```python
from build123d import *

# Parameters (mm, degrees)
SKETCH1_R                   = 30
SKETCH1_R_2                 = 15
BOSS_EXTRUDE1_DEPTH         = 17
SKETCH1_3_R                 = 15
CUT_EXTRUDE1_DEPTH          = 15
M6_TAPPED_HOLE1_D           = 5
M6_TAPPED_HOLE1_DEPTH       = 9
M6_TAPPED_HOLE1_CSINK_D     = 6.05
M6_TAPPED_HOLE1_CSINK_ANGLE = 90
M6_TAPPED_HOLE1_TIP         = 1.502151548


with BuildPart() as part:
    # Sketch1 → Boss-Extrude1 (new body)
    with BuildSketch(Plane.XY):
        Circle(SKETCH1_R)
        Circle(SKETCH1_R_2, mode=Mode.SUBTRACT)
        Circle(SKETCH1_R_2)
    extrude(amount=BOSS_EXTRUDE1_DEPTH)

    # Sketch1_3 → Cut-Extrude1 (cut)
    with BuildSketch(Plane.XY):
        Circle(SKETCH1_3_R)
    extrude(amount=CUT_EXTRUDE1_DEPTH, mode=Mode.SUBTRACT)

    # M6 Tapped Hole1
    with Locations(Plane.XY.offset(17)):
        with Locations((0, -22.5), (22.5, 0), (0, 22.5), (-22.5, 0)):
            CounterSinkHole(M6_TAPPED_HOLE1_D / 2, M6_TAPPED_HOLE1_CSINK_D / 2, depth=M6_TAPPED_HOLE1_DEPTH, counter_sink_angle=M6_TAPPED_HOLE1_CSINK_ANGLE)
            with Locations((0, 0, -(M6_TAPPED_HOLE1_DEPTH + M6_TAPPED_HOLE1_TIP / 2))):  # 118° drill point
                Cone(0, M6_TAPPED_HOLE1_D / 2, M6_TAPPED_HOLE1_TIP, mode=Mode.SUBTRACT)


solid = part.part
```
Here's how the part is built. I have some questions about the finished solid (model axes, mm). A direction names the side the tool comes from. Round coordinates to 2 decimals unless told otherwise and drop trailing zeros. Order: outer loops, then holes, each group sorted by start corner. A loop starts at its lowest first (then second) coordinate and runs counter-clockwise, first axis right, second up. Notation, with made-up numbers: M -16.5,-29.5 L 6.5,-29.5 A11 cw 6.5,-16.5 Z; hole C -6.5,13 d8. An arc over 180 degrees is marked long. One line per question, with ' | ' between items.
1) If we mould it in two halves opening along Y, with no side actions, what happens to faces 4 (the face through (-29.97, 1.32, 8.38)), 5 (the face through (0, 0, 17)), 6 (the face through (0.4, -22.67, 6.76)), 7 (the face through (0, -20, 12))? For each: +Y half, -Y half, draft (parallel to the pull), parting line (faces both ways), or undercut.
Working result:
face 4: parting line | face 5: draft | face 6: undercut | face 7: undercut
2) I need wall thicknesses on line 1 along Y through (x, z) = (0, 12); line 2 along Y through (x, z) = (-0.5, 6.25); line 3 along Z through (x, y) = (11, 4). Which ranges of each line are inside material? Lowest first, please.
Working result:
line 1: -30 to -25, -20 to -15, 15 to 20, 25 to 30 | line 2: -30 to -14.99, 14.99 to 30 | line 3: 15 to 17
3) I want a section at B-B, the plane z = 2.25. Write out the boundary of the cut face in (x, y), then the cut area to 3 significant figures.
Working result:
outline: C 0,0 d60; hole C 0,0 d30 | area: 2,120 mm²
4) For pin 1 Ø1.5 at (y, z) = (20, 5.5) entering from +X; pin 2 Ø8 at (x, z) = (9, 4.5) entering from +Y; pin 3 Ø1 at (y, z) = (-14.5, 4) entering from +X, each with a flat end and sliding along its axis, tell me the tip position at first contact or that it passes through.
Working result:
pin 1: x = 23.01 | pin 2: y = 29.58 | pin 3: x = 26.53
5) I want a section at A-A, the plane z = 15.75. Write out the boundary of the cut face in (x, y), then the cut area to 3 significant figures.
Working result:
outline: C 0,0 d60; hole C -22.5,0 d5; hole C 0,-22.5 d5; hole C 0,22.5 d5; hole C 22.5,0 d5 | area: 2,750 mm²
6) I want a section at C-C, the plane y = 13.5. Write out the boundary of the cut face in (x, z).
Working result:
outline: M -26.79,0 L -6.54,0 L -6.54,15 L 6.54,15 L 6.54,0 L 26.79,0 L 26.79,17 L -26.79,17 Z
7) For faces 1 (the face through (6, 14, 0)), 2 (the face through (0, 0, 15)), 3 (the face through (0, 25, 12)), which set-ups out of +Z, -Z, +X, -X, +Y, -Y let a thin tool reach every point of the face, with its end or its side?
Working result:
face 1: -Z, +X, -X, +Y, -Y | face 2: -Z | face 3: +Z
8) I want a section at D-D, the plane x = 17.5. Write out the boundary of the cut face in (y, z).
Working result:
outline: M -24.37,0 L 24.37,0 L 24.37,17 L -24.37,17 Z
